Source: three-view drawing plus pictorial views. Frame: mm from the lowest corner of the part. A direction names the side the tool comes from. Give positions to 0.01 mm unless a question says otherwise; leave off trailing zeros. Loops run counter-clockwise (first coordinate to the right, second up) from the corner with the lowest first, then second, coordinate; pieces in that order, holes last. Notation, with made-up numbers: (80, 9.5) - (134, 9.5) arc R17 ccw to (134, 18.5) - close; hole circle Ø6 at (-2.75, 20.25). An arc over 180 degrees is marked (long way). Answer in a Markdown table with one row per item.
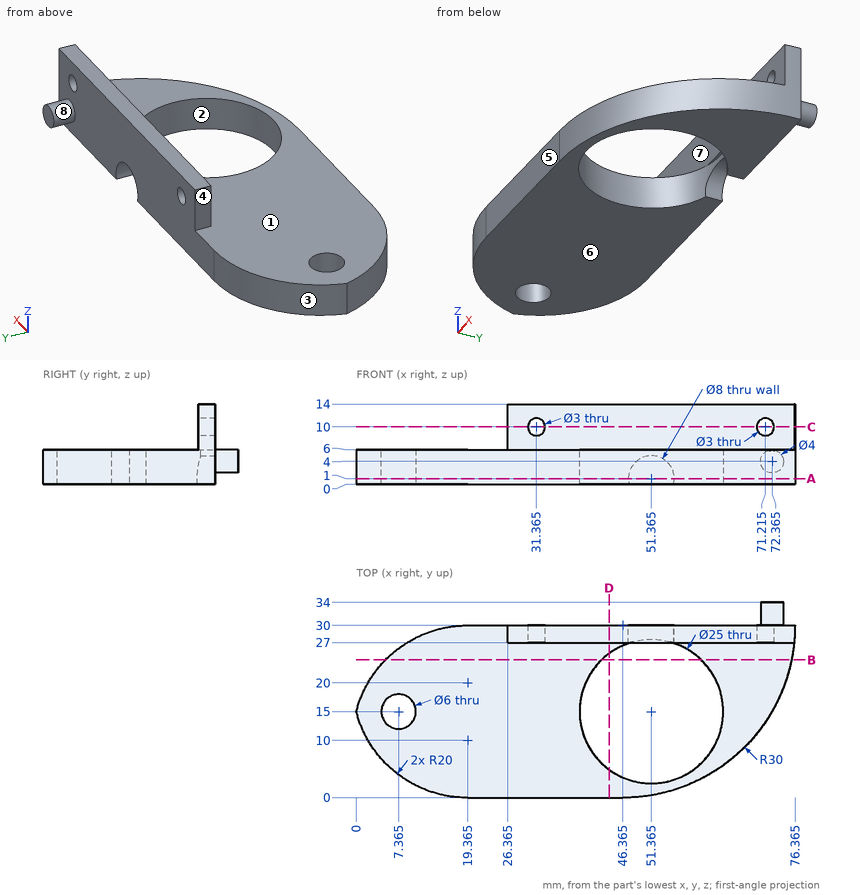
Q1. First-contact query: pin 1 (4 mm diameter, centred on x = 71.21, z = 10, fed in from -Y); pin 2 (5 mm diameter, centred on y = 24.5, z = 2.5, fed in from +X) (1 decimal); pin 3 (0.9 mm diameter, centred on y = 28.5, z = 9.5, fed in from -X) (1 decimal); pin 4 (3.5 mm diameter, centred on x = 7.36, y = 15, fed in from -Z). Flat tips, straight axial feed; report the tip coordinate or a pass-through.
Check values:
| item | result |
|---|---|
| pin 1 | y = 27 |
| pin 2 | x = 76.2 |
| pin 3 | x = 26.4 |
| pin 4 | through |
Q2. Material intervals for line 1 along Y through (x, z) = (27, 9); line 2 along Z through (x, y) = (69.5, 23); line 3 along X through (y, z) = (29.5, 9.75) (1 decimal), sorted ascending.
Check values:
| item | result |
|---|---|
| line 1 | 27 to 30 |
| line 2 | 0 to 6 |
| line 3 | 26.4 to 29.9, 32.8 to 69.7, 72.7 to 76.4 |
Q3. Draft query along Y for the marked faces 1, 2 and 3. Return one class per face: pulls with the +Y half, pulls with the -Y half, needs draft (parallel to the pull), parting line crosses it, or undercut.
Check values:
| item | result |
|---|---|
| face 1 | needs draft |
| face 2 | undercut |
| face 3 | pulls with the +Y half |
Q4. Cut plane D-D (x = 44). Output: boundary loops of the cut face in (y, z).
Check values:
| item | result |
|---|---|
| outline | (0, 0) - (4.9, 0) - (4.9, 6) - (0, 6) - close; (25.1, 0) - (30, 0) - (30, 14) - (27, 14) - (27, 6) - (25.1, 6) - close |
Q5. Cut plane C-C (z = 10). Output: boundary loops of the cut face in (x, y) (1 decimal).
Check values:
| item | result |
|---|---|
| outline | (26.4, 27) - (29.9, 27) - (29.9, 30) - (26.4, 30) - close; (32.9, 27) - (69.7, 27) - (69.7, 30) - (32.9, 30) - close; (72.7, 27) - (76.2, 27) arc R30 ccw to (76.4, 30) - (72.7, 30) - close |
Q6. Cut plane A-A (z = 1). Output: boundary loops of the cut face in (x, y) (1 decimal), and give its area (3 significant figures).
Check values:
| item | result |
|---|---|
| outline | (0, 15) arc R20 ccw to (19.4, 0) - (46.4, 0) arc R30 ccw to (76.4, 30) - (55.4, 30) - (55.4, 26.8) arc R12.5 cw (long way) to (47.4, 26.8) - (47.4, 30) - (19.4, 30) arc R20 ccw to start; hole circle Ø6 at (7.4, 15) |
| area | 1,410 mm² |
Q7. Cut plane B-B (y = 24). Output: boundary loops of the cut face in (x, z).
Check values:
| item | result |
|---|---|
| outline | (5.08, 0) - (42.69, 0) - (42.69, 6) - (5.08, 6) - close; (60.04, 0) - (75.76, 0) - (75.76, 6) - (60.04, 6) - close |
Q8. Reachability of the marked faces 4, 5, 6, 7 and 8 from +Z, -Z, +X, -X, +Y, -Y: full face, straight path, thin tool, end or side. Return the list, or none.
Check values:
| item | result |
|---|---|
| face 4 | +Z, -X, +Y, -Y |
| face 5 | +Z, -Z, +X, -X, -Y |
| face 6 | -Z, +X, -X, +Y, -Y |
| face 7 | +Z, +X, -X, -Y |
| face 8 | +Y |
